Geometry check sheet. Reference: the model listing, model coordinates, mm. Face numbers are marked on the shaded views. A direction names the side the tool comes from. Round coordinates to 2 decimals unless told otherwise and drop trailing zeros. Write each loop counter-clockwise with the first axis right and the second up, starting at its lowest first coordinate (ties: lowest second). Pieces come first, ordered by that corner, then holes.
Item 1: Cross-section at C-C (z = 0). Enter the section's corners in (x, y).
Item 2: Scan lines: probe 1 along Z at (x, y) = (-0.25, 5); probe 2 along Z at (x, y) = (0, 6.5); probe 3 along Y at (x, z) = (3, 6). Record each from-to range of solid material in increasing order.
Item 3: Access from +Z, -Z, +X, -X, +Y, -Y to the whole of each face (thin tool, end or side, straight path). Record for the marked faces 1 and 2.
Item 4: Cross-section at A-A (x = -1.5). Enter the section's corners in (y, z).
Item 5: Cross-section at B-B (y = 5.5). Enter the section's corners in (x, z), then the cut area to 3 significant figures.
Item 6: Depth check by flat-ended pin: P1, Ø4, axis at y = 5.5, z = 5.5, coming from the +X side; P2, Ø2.5, axis at y = 5.5, z = -5.5, coming from the -X side; P3, Ø3, axis at x = -1.5, y = 10.5, coming from the -Z side; P4, Ø1, axis at x = 0, y = 8.5, coming from the +Z side. Enter the tip coordinate at first touch or a pass-through.
Item 7: Draft check along Y on the marked faces 3, 4 and 5. Enter one of: pulls with the +Y half, pulls with the -Y half, needs draft (parallel to the pull), parting line crosses it, or undercut.
Item 8: Cross-section at D-D (x = -2.75). Enter the section's corners in (y, z).
from build123d import *

# Parameters (mm, degrees)
ESQUISSE1_R             = 4
ESQUISSE1_R_2           = 2
BOSS_EXTRU_1_DEPTH      = 13.5
BOSS_EXTRU_2_REACH      = 30.137
BOSS_EXTRU_2_END_RADIUS = 4
BOSS_EXTRU_2_START      = 13.5
ESQUISSE2_R             = 4
ESQUISSE2_R_2           = 2
ESQUISSE3_R             = 2.35
ESQUISSE3_R_2           = 1.6
BOSS_EXTRU_3_DEPTH      = 4


with BuildPart() as part:
    # Esquisse1 → Boss.-Extru.1 (new, symmetric)
    with BuildSketch(Plane.XY):
        Circle(ESQUISSE1_R)
        Circle(ESQUISSE1_R_2, mode=Mode.SUBTRACT)
    extrude(amount=BOSS_EXTRU_1_DEPTH, both=True)

    # Boss.-Extru.2: up to this cylinder (the profile starts outside it)
    boss_extru_2_end = Plane(origin=(0, 0, -3.886863), z_dir=(0, 0, -1)) * Cylinder(BOSS_EXTRU_2_END_RADIUS, 69.274, mode=Mode.PRIVATE)
    # Esquisse2 → Boss.-Extru.2 (add, up to the surface)
    with BuildSketch(Plane(origin=(0, 0, 0), x_dir=(1, 0, 0), z_dir=(0, 1, 0)).offset(BOSS_EXTRU_2_START), mode=Mode.PRIVATE) as boss_extru_2_sk1:
        with Locations(Location((0, 0, 0), (0, 0, 270))):
            Circle(ESQUISSE2_R)
        with Locations(Location((0, 0, 0), (0, 0, 270))):
            Circle(ESQUISSE2_R_2, mode=Mode.SUBTRACT)
    boss_extru_2_tool1 = extrude(boss_extru_2_sk1.sketch, amount=-BOSS_EXTRU_2_REACH, mode=Mode.PRIVATE) - boss_extru_2_end
    add(boss_extru_2_tool1.solids().sort_by_distance((0, 13.5, -3.886863))[0])

    # Esquisse3 → Boss.-Extru.3 (add, symmetric)
    # profile 1 of 2: a face of its own
    with BuildSketch(Plane(origin=(0, 0, 0), x_dir=(0, 0, -1), z_dir=(1, 0, 0))):
        with Locations((-5.5, 5.5)):
            Circle(ESQUISSE3_R)
        with Locations((-5.5, 5.5)):
            Circle(ESQUISSE3_R_2, mode=Mode.SUBTRACT)
    # profile 2 of 2: a face of its own
    with BuildSketch(Plane(origin=(0, 0, 0), x_dir=(0, 0, -1), z_dir=(1, 0, 0))):
        with Locations(Location((5.5, 5.5, 0), (0, 0, 180))):
            Circle(ESQUISSE3_R)
        with Locations(Location((5.5, 5.5, 0), (0, 0, 180))):
            Circle(ESQUISSE3_R_2, mode=Mode.SUBTRACT)
    extrude(amount=BOSS_EXTRU_3_DEPTH, both=True)


solid = part.part
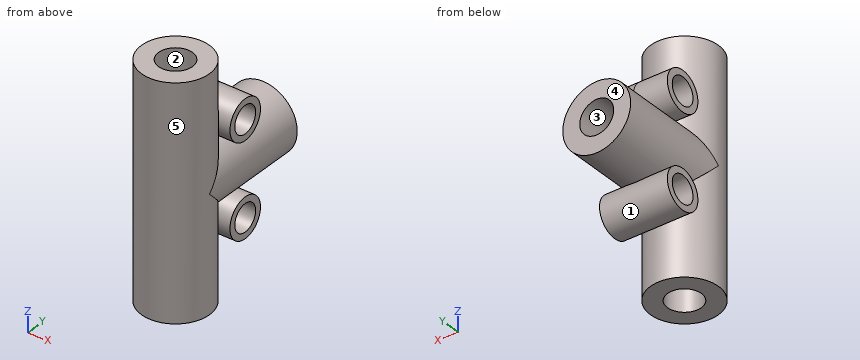
Resolved:
1. outline: (-4, 0) arc R4 ccw to (4, 0) - (4, 13.5) - (2, 13.5) - (2, 3.46) arc R4 ccw to (-2, 3.46) - (-2, 13.5) - (-4, 13.5) - close; hole circle Ø4 at (0, 0)
2. probe 1: z = -7.8 to -7.02, -3.99 to -1.98, 1.98 to 3.99, 7.02 to 7.8
2. probe 2: z = -7.63 to -6.75, -4.25 to -2, 2 to 4.25, 6.75 to 7.63
2. probe 3: y = -2.65 to 2.65, 3.2 to 3.98, 7.02 to 7.8
3. face 1: none
3. face 2: +Z, -Z
4. outline: (-3.71, -13.5) - (-1.32, -13.5) - (-1.32, 13.5) - (-3.71, 13.5) - close; (1.32, -13.5) - (3.71, -13.5) - (3.71, -7.02) arc R2.35 ccw (long way) to (7.02, -3.71) - (13.5, -3.71) - (13.5, -1.32) - (3.71, -1.32) - (3.71, 1.32) - (13.5, 1.32) - (13.5, 3.71) - (7.02, 3.71) arc R2.35 ccw (long way) to (3.71, 7.02) - (3.71, 13.5) - (1.32, 13.5) - close; hole (3.71, -3.98) arc R2.35 cw to (3.98, -3.71) - (3.71, -3.71) - close; hole (3.71, 3.71) - (3.98, 3.71) arc R2.35 cw to (3.71, 3.98) - close; hole circle Ø3.2 at (5.5, -5.5); hole circle Ø3.2 at (5.5, 5.5)
5. outline: (-4, -7.85) - (4, -7.85) - (4, -7.1) - (-4, -7.1) - close; (-4, -3.9) - (-0.89, -3.9) arc R4 ccw to (0.89, -3.9) - (4, -3.9) - (4, -3.15) - (2.47, -3.15) arc R4 ccw to (2.47, 3.15) - (4, 3.15) - (4, 3.9) - (0.89, 3.9) arc R4 ccw to (-0.89, 3.9) - (-4, 3.9) - (-4, 3.15) - (-2.47, 3.15) arc R4 ccw to (-2.47, -3.15) - (-4, -3.15) - close; (-4, 7.1) - (4, 7.1) - (4, 7.85) - (-4, 7.85) - close; hole circle Ø4 at (0, 0)
5. area: 56.2 mm2
6. P1: stops at x = 4
6. P2: passes through
6. P3: stops at z = -4
6. P4: stops at z = 4
7. face 3: needs draft
7. face 4: pulls with the +Y half
7. face 5: undercut
8. outline: (-2.9, -13.5) - (2.9, -13.5) - (2.9, -2.9) - (13.5, -2.9) - (13.5, 2.9) - (2.9, 2.9) - (2.9, 13.5) - (-2.9, 13.5) - close; circle Ø4.7 at (5.5, -5.5); circle Ø4.7 at (5.5, 5.5); hole circle Ø3.2 at (5.5, -5.5); hole circle Ø3.2 at (5.5, 5.5)
